from build123d import *

# Parameters (mm, degrees)
SKETCH1_W           = 180
SKETCH1_H           = 50
BOSS_EXTRUDE1_DEPTH = 6
SKETCH2_R           = 5.25
CUT_EXTRUDE1_DEPTH  = 7
FILLET1_R           = 10
SKETCH3_W           = 5
SKETCH3_H           = 20
SKETCH3_W_2         = 10
SKETCH3_H_2         = 5
CUT_EXTRUDE2_DEPTH  = 7


with BuildPart() as part:
    # Sketch1 → Boss-Extrude1 (new body)
    with BuildSketch(Plane.XY):
        Rectangle(SKETCH1_W, SKETCH1_H)
    extrude(amount=BOSS_EXTRUDE1_DEPTH)

    # Sketch2 → Cut-Extrude1 (cut, through all)
    with BuildSketch(Plane.XY.offset(6)):
        with Locations((-64.05, 5)):
            Circle(SKETCH2_R)
        with Locations((4.15, 5)):
            Circle(SKETCH2_R)
        with Locations((71.05, 5)):
            Circle(SKETCH2_R)
    extrude(amount=-CUT_EXTRUDE1_DEPTH, mode=Mode.SUBTRACT)

    # Fillet1
    fillet1_edges = [part.edges().sort_by_distance(p)[0] for p in [
        (-90, 25, 3),
        (90, 25, 3),
    ]]
    fillet(fillet1_edges, radius=FILLET1_R)

    # Sketch3 → Cut-Extrude2 (cut, through all)
    with BuildSketch(Plane(origin=(0, 0, 0), x_dir=(-1, 0, 0), z_dir=(0, 0, -1))):
        with Locations((-71.05, -15)):
            Rectangle(SKETCH3_W, SKETCH3_H)
        with Locations((64.05, -15)):
            Rectangle(SKETCH3_W, SKETCH3_H)
        with Locations((-71.05, -13)):
            Rectangle(SKETCH3_W_2, SKETCH3_H_2)
        with Locations((64.05, -13)):
            Rectangle(SKETCH3_W_2, SKETCH3_H_2)
    extrude(amount=-CUT_EXTRUDE2_DEPTH, mode=Mode.SUBTRACT)


solid = part.part
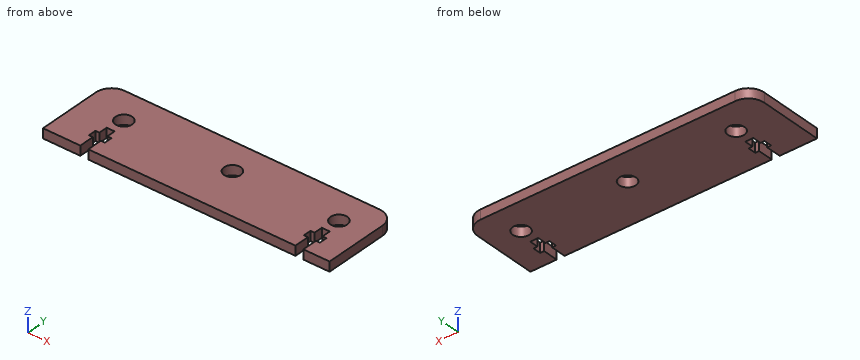
Source: CAD feature listing. Evaluate the final solid. Frame: model axes, mm. Round coordinates to 2 decimals unless told otherwise and drop trailing zeros. Loops run counter-clockwise (first coordinate to the right, second up) from the corner with the lowest first, then second, coordinate; pieces in that order, holes last. Notation, with made-up numbers: (67.5, -36.75) - (94.5, -36.75) arc R18 ccw to (94.5, -25.75) - close; hole circle Ø3 at (46.5, -20.5). An arc over 180 degrees is marked (long way). Write item = value, one per line. Start each with the question number.
Item 1: Section query A-A on x = -64.05. Output: boundary loops of the cut face in (y, z).
Item 2: First-contact query: pin 1 Ø8.5 at (x, y) = (-64.05, 5) entering from +Z; pin 2 Ø1.5 at (x, z) = (-63, 3.5) entering from -Y. Flat tips, straight axial feed; report the tip coordinate or a pass-through.
Item 3: Material intervals for line 1 (X direction, y = -8.5, z = 0.5); line 2 (X direction, y = 2, z = 1.9); line 3 (Y direction, x = 71.05, z = 4.8), sorted ascending.
Item 4: Section query B-B on z = 4.15. Count the separate pieces of the cut face and the enclosed holes in it, plus the area to 3 significant figures.
Item 5: Section query D-D on y = 5. Output: boundary loops of the cut face in (x, z), plus the area to 3 significant figures.
Item 6: Section query C-C on y = -17. Output: boundary loops of the cut face in (x, z).
Results list:
q1.outline = (-5, 0) - (-0.25, 0) - (-0.25, 6) - (-5, 6) - close; (10.25, 0) - (25, 0) - (25, 6) - (10.25, 6) - close
q2.pin_1 = through
q2.pin_2 = -5
q3.line_1 = -90 to -66.55, -61.55 to 68.55, 73.55 to 90
q3.line_2 = -90 to -68.36, -59.74 to -0.16, 8.46 to 66.74, 75.36 to 90
q3.line_3 = -5 to -0.25, 10.25 to 25
q4.separate_pieces = 1
q4.enclosed_holes = 3
q4.area = 8,450 mm²
q5.outline = (-90, 0) - (-69.3, 0) - (-69.3, 6) - (-90, 6) - close; (-58.8, 0) - (-1.1, 0) - (-1.1, 6) - (-58.8, 6) - close; (9.4, 0) - (65.8, 0) - (65.8, 6) - (9.4, 6) - close; (76.3, 0) - (90, 0) - (90, 6) - (76.3, 6) - close
q5.area = 891 mm²
q6.outline = (-90, 0) - (-66.55, 0) - (-66.55, 6) - (-90, 6) - close; (-61.55, 0) - (68.55, 0) - (68.55, 6) - (-61.55, 6) - close; (73.55, 0) - (90, 0) - (90, 6) - (73.55, 6) - close
